Source: CAD feature listing. Evaluate the final solid. Frame: model axes, mm. Coordinates: 2 decimals unless noted, no trailing zeros. Loops run counter-clockwise (first coordinate to the right, second up) from the corner with the lowest first, then second, coordinate; pieces in that order, holes last. Notation, with made-up numbers: (-7.75, 12.25) -> (42.25, 12.25) arc R27 cw to (42.25, 46.25) -> close; hole circle Ø11 at (77.25, 62). An arc over 180 degrees is marked (long way). Answer as a JSON object with one key per item and string values. Group by question number.
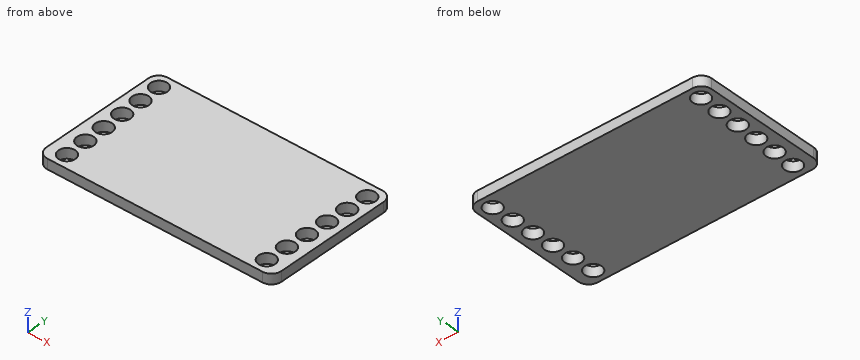
from build123d import *

# Parameters (mm, degrees)
SKETCH1_W           = 70
SKETCH1_H           = 40.5
SKETCH1_R           = 2.5
BOSS_EXTRUDE1_DEPTH = 3
FILLET1_R           = 3


with BuildPart() as part:
    # Sketch1 → Boss-Extrude1 (new body)
    with BuildSketch(Plane.XY):
        with Locations((0, 19.75)):
            Rectangle(SKETCH1_W, SKETCH1_H)
        with Locations((-29.75, 3.5)):
            Circle(SKETCH1_R, mode=Mode.SUBTRACT)
        with Locations((-30, 10)):
            Circle(SKETCH1_R, mode=Mode.SUBTRACT)
        with Locations((-30.25, 16.5)):
            Circle(SKETCH1_R, mode=Mode.SUBTRACT)
        with Locations((-30.5, 23)):
            Circle(SKETCH1_R, mode=Mode.SUBTRACT)
        with Locations((-30.75, 29.5)):
            Circle(SKETCH1_R, mode=Mode.SUBTRACT)
        with Locations((-31, 36)):
            Circle(SKETCH1_R, mode=Mode.SUBTRACT)
        with Locations((29.75, 3.5)):
            Circle(SKETCH1_R, mode=Mode.SUBTRACT)
        with Locations((30, 10)):
            Circle(SKETCH1_R, mode=Mode.SUBTRACT)
        with Locations((30.25, 16.5)):
            Circle(SKETCH1_R, mode=Mode.SUBTRACT)
        with Locations((30.5, 23)):
            Circle(SKETCH1_R, mode=Mode.SUBTRACT)
        with Locations((30.75, 29.5)):
            Circle(SKETCH1_R, mode=Mode.SUBTRACT)
        with Locations((31, 36)):
            Circle(SKETCH1_R, mode=Mode.SUBTRACT)
    extrude(amount=BOSS_EXTRUDE1_DEPTH)

    # Fillet1
    fillet1_edges = [part.edges().sort_by_distance(p)[0] for p in [
        (-35, 40, 1.5),
        (35, 40, 1.5),
        (35, -0.5, 1.5),
        (-35, -0.5, 1.5),
    ]]
    fillet(fillet1_edges, radius=FILLET1_R)


solid = part.part
1. Ray query, L1, parallel to X at y = 24.5, z = 0.45; L2, parallel to X at y = 5, z = 2.85. Return the intervals inside material, ascending.
2. Pin query (flat end, axial travel): pin 1 Ø4.5 at (x, y) = (-30.25, 16.5) entering from +Z. Return the tip coordinate at first contact, or that it passes through.
3. Section query B-B on y = 23. Return loops of the section in (x, z).
4. Section query C-C on x = -30.25. Return loops of the section in (y, z), then the cut area to 3 significant figures.
5. Section query A-A on z = 1.05. State how many separate pieces and enclosed holes the cut face has, then the cut area to 3 significant figures.
6. Section query D-D on x = 29.75. Return loops of the section in (y, z), then the cut area to 3 significant figures.
Solved:
{
 "1": {"L1": "-35 to -32.5, -28.5 to 28.5, 32.5 to 35", "L2": "-35 to -31.75, -27.75 to 27.75, 31.75 to 35"},
 "2": {"pin 1": "through"},
 "3": {"outline": "(-35, 0) -> (-33, 0) -> (-33, 3) -> (-35, 3) -> close; (-28, 0) -> (28, 0) -> (28, 3) -> (-28, 3) -> close; (33, 0) -> (35, 0) -> (35, 3) -> (33, 3) -> close"},
 "4": {"outline": "(-0.5, 0) -> (1.05, 0) -> (1.05, 3) -> (-0.5, 3) -> close; (5.95, 0) -> (7.51, 0) -> (7.51, 3) -> (5.95, 3) -> close; (12.49, 0) -> (14, 0) -> (14, 3) -> (12.49, 3) -> close; (19, 0) -> (20.51, 0) -> (20.51, 3) -> (19, 3) -> close; (25.49, 0) -> (27.05, 0) -> (27.05, 3) -> (25.49, 3) -> close; (31.95, 0) -> (33.62, 0) -> (33.62, 3) -> (31.95, 3) -> close; (38.38, 0) -> (40, 0) -> (40, 3) -> (38.38, 3) -> close", "area": "32.9 mm^2"},
 "5": {"separate pieces": "1", "enclosed holes": "12", "area": "2,590 mm^2"},
 "6": {"outline": "(-0.5, 0) -> (1, 0) -> (1, 3) -> (-0.5, 3) -> close; (6, 0) -> (7.51, 0) -> (7.51, 3) -> (6, 3) -> close; (12.49, 0) -> (14.05, 0) -> (14.05, 3) -> (12.49, 3) -> close; (18.95, 0) -> (20.62, 0) -> (20.62, 3) -> (18.95, 3) -> close; (25.38, 0) -> (27.21, 0) -> (27.21, 3) -> (25.38, 3) -> close; (31.79, 0) -> (33.83, 0) -> (33.83, 3) -> (31.79, 3) -> close; (38.17, 0) -> (40, 0) -> (40, 3) -> (38.17, 3) -> close", "area": "35.8 mm^2"}
}
